Geometry: final body of the model. Coordinates: model frame, mm. A direction names the side the tool comes from. Give positions to 0.01 mm unless a question says otherwise; leave off trailing zeros. Loops run counter-clockwise (first coordinate to the right, second up) from the corner with the lowest first, then second, coordinate; pieces in that order, holes last.
1. First-contact query: P1, Ø3, axis at y = 3.5, z = 5, coming from the +X side; P2, Ø0.8, axis at y = 6, z = 9, coming from the +X side; P3, Ø2, axis at x = 15, z = 5.5, coming from the +Y side. Flat tips, straight axial feed; report the tip coordinate or a pass-through.
2. Section B-B, the plane z = 1. Output: boundary loops of the cut face in (x, y), then the cut area to 3 significant figures.
3. Material intervals for line 1 along Y through (x, z) = (10, 9.25); line 2 along Y through (x, z) = (17.5, 2.25); line 3 along Z through (x, y) = (2, -3.05), sorted ascending.
4. Access query for faces 5 (the face through (-2, 0, 2)), 6 (the face through (-4, 5, 6)), 7 (the face through (13, 0, 7)), 8 (the face through (2, 4, 10.47)), 9 (the face through (14.935, -1.452, 11.493)). Directions: +Z, -Z, +X, -X, +Y, -Y. A direction counts if a zero-diameter tool reaches every point of the face in a straight line with its end or side. Return the directions, or none.
5. Draft query along Z for faces 1 (the face through (2, -4, 10.47)), 2 (the face through (20.04, -1.496, 11.493)), 3 (the face through (4, 2.55, 7)), 4 (the face through (1.04, 3.51, 9.98)). Return one class per face: +Z half, -Z half, draft (parallel to the pull), parting line (faces both ways), or undercut.
6. Section A-A, the plane z = 8.5. Output: boundary loops of the cut face in (x, y), then the cut area to 3 significant figures.
7. Section C-C, the plane x = 10.5. Output: boundary loops of the cut face in (y, z), then the cut area to 3 significant figures.
8. Section D-D, the plane x = 1. Output: boundary loops of the cut face in (y, z), then the cut area to 3 significant figures.
from build123d import *

# Parameters (mm, degrees)
SKETCH1_R           = 1.65
BOSS_EXTRUDE1_DEPTH = 12
SKETCH2_W           = 17
SKETCH2_H           = 5.1
CUT_EXTRUDE1_DEPTH  = 9
CUT_EXTRUDE2_DEPTH  = 3
CHAMFER1_SIZE       = 0.4
CHAMFER1_SIZE2      = 1
CHAMFER2_SIZE       = 0.3
CUT_EXTRUDE3_DEPTH  = 12.5
CUT_EXTRUDE4_DEPTH  = 2.5
SKETCH6_W           = 2
SKETCH6_H           = 5.1
CUT_EXTRUDE5_DEPTH  = 4


with BuildPart() as part:
    # Sketch1 → Boss-Extrude1 (new body)
    with BuildSketch(Plane.XY):
        with BuildLine():
            Line((-4, 7), (-4, -4.5))
            Line((-4, -4.5), (17.5, -4.5))
            ThreePointArc((17.5, -4.5), (22, 0), (17.5, 4.5))
            Line((17.5, 4.5), (13, 4.5))
            Line((13, 4.5), (13, 7))
            Line((13, 7), (-4, 7))
        make_face()
        with Locations((17.5, 0)):
            Circle(SKETCH1_R, mode=Mode.SUBTRACT)
    extrude(amount=BOSS_EXTRUDE1_DEPTH)

    # Sketch2 → Cut-Extrude1 (cut)
    with BuildSketch(Plane.XY.offset(12)):
        with Locations((4.5, 0)):
            Rectangle(SKETCH2_W, SKETCH2_H)
    extrude(amount=-CUT_EXTRUDE1_DEPTH, mode=Mode.SUBTRACT)

    # Sketch3 → Cut-Extrude2 (cut)
    with BuildSketch(Plane.XY.offset(12)):
        Polygon((14.324573519, 0), (15.91228676, -2.75), (19.08771324, -2.75), (20.675426481, 0), (19.08771324, 2.75), (15.91228676, 2.75), align=None)
    extrude(amount=-CUT_EXTRUDE2_DEPTH, mode=Mode.SUBTRACT)

    # Chamfer1
    chamfer1_edges = [part.edges().sort_by_distance(p)[0] for p in [
        (4.5, -2.55, 12),
        (13, 0, 12),
        (4.5, 2.55, 12),
        (15.11843014, 1.375, 12),
        (15.11843014, -1.375, 12),
        (17.5, -2.75, 12),
        (19.88156986, -1.375, 12),
        (19.88156986, 1.375, 12),
        (17.5, 2.75, 12),
    ]]
    chamfer1_side = [part.faces().sort_by_distance(p)[0] for p in [
        (4.5, 6.71570262, 12),
    ]]
    chamfer(chamfer1_edges, length=CHAMFER1_SIZE, length2=CHAMFER1_SIZE2, reference=chamfer1_side[0])

    # Chamfer2
    chamfer2_edges = [part.edges().sort_by_distance(p)[0] for p in [
        (15.85, 0, 0),
        (22, 0, 0),
        (6.75, -4.5, 0),
        (-4, 1.25, 0),
        (4.5, 7, 0),
        (13, 5.75, 0),
        (15.25, 4.5, 0),
    ]]
    chamfer(chamfer2_edges, length=CHAMFER2_SIZE)

    # Sketch4 → Cut-Extrude3 (cut, through all)
    with BuildSketch(Plane(origin=(0, -4.5, 0), x_dir=(1, 0, 0), z_dir=(0, 1, 0))):
        with BuildLine():
            Line((3.329547877, -9.477139931), (2.599853793, -10.47))
            Line((2.599853793, -10.47), (1.400146207, -10.47))
            Line((1.400146207, -10.47), (0.670452123, -9.477139931))
            ThreePointArc((0.670452123, -9.477139931), (2, -6.85), (3.329547877, -9.477139931))
        make_face()
    extrude(amount=CUT_EXTRUDE3_DEPTH, mode=Mode.SUBTRACT)

    # Sketch5 → Cut-Extrude4 (cut)
    with BuildSketch(Plane(origin=(0, 7, 0), x_dir=(1, 0, 0), z_dir=(0, 1, 0))):
        Polygon((-0.8, -12), (4.8, -12), (4.8, -6.883419246), (2, -5.266838493), (-0.8, -6.883419246), align=None)
    extrude(amount=-CUT_EXTRUDE4_DEPTH, mode=Mode.SUBTRACT)

    # Sketch6 → Cut-Extrude5 (cut, through all)
    with BuildSketch(Plane.XY.offset(3)):
        with Locations((-3, 0)):
            Rectangle(SKETCH6_W, SKETCH6_H)
    extrude(amount=-CUT_EXTRUDE5_DEPTH, mode=Mode.SUBTRACT)


solid = part.part
Answers below:
1. P1: stops at x = 21.53
1. P2: stops at x = 13
1. P3: stops at y = 4.5
2. outline: (-4, -4.5) - (17.5, -4.5) arc R4.5 ccw to (17.5, 4.5) - (13, 4.5) - (13, 7) - (-4, 7) - (-4, 2.55) - (-2, 2.55) - (-2, -2.55) - (-4, -2.55) - close; hole circle Ø3.3 at (17.5, 0)
2. area: 249 mm2
3. line 1: y = -4.5 to -2.55, 2.55 to 7
3. line 2: y = -4.5 to -1.65, 1.65 to 4.5
3. line 3: z = 0 to 6.85, 10.47 to 12
4. face 5: +Z, -Z, -X
4. face 6: +Z, -Z, -X, +Y, -Y
4. face 7: +Z, -X
4. face 8: +Y, -Y
4. face 9: +Z
5. face 1: undercut
5. face 2: +Z half
5. face 3: draft
5. face 4: undercut
6. outline: (-4, -4.5) - (0.35, -4.5) - (0.35, -2.55) - (-4, -2.55) - close; (-4, 2.55) - (0.35, 2.55) - (0.35, 4.5) - (-0.8, 4.5) - (-0.8, 7) - (-4, 7) - close; (3.65, -4.5) - (17.5, -4.5) arc R4.5 ccw to (17.5, 4.5) - (13, 4.5) - (13, 7) - (4.8, 7) - (4.8, 4.5) - (3.65, 4.5) - (3.65, 2.55) - (13, 2.55) - (13, -2.55) - (3.65, -2.55) - close; hole circle Ø3.3 at (17.5, 0)
6. area: 146 mm2
7. outline: (-4.5, 0.3) - (-4.2, 0) - (6.7, 0) - (7, 0.3) - (7, 12) - (2.95, 12) - (2.55, 11) - (2.55, 3) - (-2.55, 3) - (-2.55, 11) - (-2.95, 12) - (-4.5, 12) - close
7. area: 91.6 mm2
8. outline: (-4.5, 0.3) - (-4.2, 0) - (6.7, 0) - (7, 0.3) - (7, 5.84) - (4.5, 5.84) - (4.5, 7.19) - (2.55, 7.19) - (2.55, 3) - (-2.55, 3) - (-2.55, 7.19) - (-4.5, 7.19) - close; (-4.5, 9.93) - (-2.55, 9.93) - (-2.55, 11) - (-2.95, 12) - (-4.5, 12) - close; (2.55, 9.93) - (4.5, 9.93) - (4.5, 12) - (2.95, 12) - (2.55, 11) - close
8. area: 65.5 mm2
